Input: part model. Units: mm. Frame: model coordinates. A direction names the side the tool comes from. Round coordinates to 2 decimals unless told otherwise and drop trailing zeros. Order: outer loops, then holes, each group sorted by start corner. A loop starts at its lowest first (then second) coordinate and runs counter-clockwise, first axis right, second up.
Item 1: Cut plane A-A on z = 6.5. Output: boundary loops of the cut face in (x, y), then the cut area to 3 significant figures.
Item 2: First-contact query: pin 1 (1.2 mm diameter, centred on y = 3, z = 5, fed in from +X); pin 2 (5 mm diameter, centred on y = 2.25, z = 5, fed in from +X); pin 3 (2 mm diameter, centred on x = 12.5, y = 9, fed in from +Z). Flat tips, straight axial feed; report the tip coordinate or a pass-through.
Item 3: Cut plane B-B on x = 10.5. Output: boundary loops of the cut face in (y, z), then the cut area to 3 significant figures.
Item 4: Cut plane D-D on z = -5.75. Output: boundary loops of the cut face in (x, y).
Item 5: Mould query, pull axis Y, two halves, no side actions, for faces 1 (the flat face through (0, 12, 0)), 2 (the flat face through (9.25, 11.5, -6.8)), 3 (the cylindrical face through (12.7, 0.71, 6.64)). Classes: released by +Y, released by -Y, zero draft, split by the parting line, or undercut.
Item 6: Reachability of faces 4 (the cylindrical face through (12.7, 11.39, 6.54)), 5 (the flat face through (9.25, 0.5, 6.8)), 6 (the flat face through (9.25, 11, 0)), 7 (the flat face through (9.25, 6, -6)), 8 (the cylindrical face through (13.487, 5.324, 6.726)) from +Z, -Z, +X, -X, +Y, -Y: full face, straight path, thin tool, end or side. Return the list, or none.
Item 7: Cut plane C-C on y = 6. Output: boundary loops of the cut face in (x, z), then the cut area to 3 significant figures.
Item 8: Line query: L1, parallel to Y at x = 16, z = -6; L2, parallel to X at y = 5.5, z = 4.25; L3, parallel to X at y = 8, z = 4.5. Output: solid intervals per line, ascending.
```python
from build123d import *

# Parameters (mm, degrees)
SKETCH_1_W      = 18.5
SKETCH_1_H      = 14.5
EXTRUDE_1_DEPTH = 12
SKETCH_2_R      = 2.25
SKETCH_2_R_2    = 2
EXTRUDE_2_DEPTH = 7
SKETCH_4_R      = 1.5
EXTRUDE_3_DEPTH = 5.5
SKETCH_6_R      = 1
EXTRUDE_4_DEPTH = 3.5


with BuildPart() as part:
    # 스케치1 → 보스-돌출1 (new body)
    with BuildSketch(Plane(origin=(0, 0, 0), x_dir=(1, 0, 0), z_dir=(0, 1, 0))):
        Rectangle(SKETCH_1_W, SKETCH_1_H)
    extrude(amount=EXTRUDE_1_DEPTH)

    # 스케치2 → 보스-돌출2 (add)
    # profile 1 of 5: a face of its own
    with BuildSketch(Plane(origin=(9.25, 0, 0), x_dir=(0, 0, -1), z_dir=(1, 0, 0))):
        with Locations((-5, 9.75)):
            Circle(SKETCH_2_R)
        with Locations((-5, 9.75)):
            Circle(SKETCH_2_R_2, mode=Mode.SUBTRACT)
    # profile 2 of 5: a face of its own
    with BuildSketch(Plane(origin=(9.25, 0, 0), x_dir=(0, 0, -1), z_dir=(1, 0, 0))):
        with BuildLine():
            Line((2.75, 9.75), (-2.75, 9.75))
            ThreePointArc((-2.75, 9.75), (-3.409009742, 8.159009742), (-5, 7.5))
            Line((-5, 7.5), (-5, 4.5))
            ThreePointArc((-5, 4.5), (-3.409009742, 3.840990258), (-2.75, 2.25))
            Line((-2.75, 2.25), (2.75, 2.25))
            ThreePointArc((2.75, 2.25), (3.409009742, 3.840990258), (5, 4.5))
            Line((5, 4.5), (5, 7.5))
            ThreePointArc((5, 7.5), (3.409009742, 8.159009742), (2.75, 9.75))
        make_face()
    # profile 3 of 5: a face of its own
    with BuildSketch(Plane(origin=(9.25, 0, 0), x_dir=(0, 0, -1), z_dir=(1, 0, 0))):
        with Locations((5, 9.75)):
            Circle(SKETCH_2_R)
        with Locations((5, 9.75)):
            Circle(SKETCH_2_R_2, mode=Mode.SUBTRACT)
    # profile 4 of 5: a face of its own
    with BuildSketch(Plane(origin=(9.25, 0, 0), x_dir=(0, 0, -1), z_dir=(1, 0, 0))):
        with Locations((5, 2.25)):
            Circle(SKETCH_2_R)
        with Locations((5, 2.25)):
            Circle(SKETCH_2_R_2, mode=Mode.SUBTRACT)
    # profile 5 of 5: a face of its own
    with BuildSketch(Plane(origin=(9.25, 0, 0), x_dir=(0, 0, -1), z_dir=(1, 0, 0))):
        with Locations((-5, 2.25)):
            Circle(SKETCH_2_R)
        with Locations((-5, 2.25)):
            Circle(SKETCH_2_R_2, mode=Mode.SUBTRACT)
    extrude(amount=EXTRUDE_2_DEPTH)

    # 스케치4 → 보스-돌출3 (add)
    with BuildSketch(Plane(origin=(16.25, 0, 0), x_dir=(0, 0, -1), z_dir=(1, 0, 0))):
        with Locations((0, 6)):
            Circle(SKETCH_4_R)
    extrude(amount=EXTRUDE_3_DEPTH)

    # 스케치6 → 보스-돌출4 (add)
    with BuildSketch(Plane.XY.offset(5)):
        with Locations(Location((12.75, 6, 0), (0, 0, 180))):
            Circle(SKETCH_6_R)
    extrude(amount=EXTRUDE_4_DEPTH)


solid = part.part
```
From the geometry:
1. outline: (-9.25, 0) - (9.25, 0) - (9.25, 0.57) - (16.25, 0.57) - (16.25, 0.93) - (9.25, 0.93) - (9.25, 3.57) - (16.25, 3.57) - (16.25, 3.93) - (9.25, 3.93) - (9.25, 8.07) - (16.25, 8.07) - (16.25, 8.43) - (9.25, 8.43) - (9.25, 11.07) - (16.25, 11.07) - (16.25, 11.43) - (9.25, 11.43) - (9.25, 12) - (-9.25, 12) - close; circle Ø2 at (12.75, 6)
1. area: 235 mm2
2. pin 1: stops at x = 9.25
2. pin 2: stops at x = 16.25
2. pin 3: stops at z = 7.25
3. outline: (2.25, -2.75) arc R2.25 ccw (long way) to (4.5, -5) - (7.5, -5) arc R2.25 ccw (long way) to (9.75, -2.75) - (9.75, 2.75) arc R2.25 ccw (long way) to (7.5, 5) - (4.5, 5) arc R2.25 ccw (long way) to (2.25, 2.75) - close; hole circle Ø4 at (2.25, -5); hole circle Ø4 at (2.25, 5); hole circle Ø4 at (9.75, -5); hole circle Ø4 at (9.75, 5)
3. area: 72.4 mm2
4. outline: (-9.25, 0) - (9.25, 0) - (9.25, 0.13) - (16.25, 0.13) - (16.25, 0.4) - (9.25, 0.4) - (9.25, 4.1) - (16.25, 4.1) - (16.25, 4.37) - (9.25, 4.37) - (9.25, 7.63) - (16.25, 7.63) - (16.25, 7.9) - (9.25, 7.9) - (9.25, 11.6) - (16.25, 11.6) - (16.25, 11.87) - (9.25, 11.87) - (9.25, 12) - (-9.25, 12) - close
5. face 1: released by +Y
5. face 2: zero draft
5. face 3: undercut
6. face 4: +X
6. face 5: +Z, +X, -Y
6. face 6: +X, +Y
6. face 7: -Z, +X
6. face 8: +Z
7. outline: (-9.25, -7.25) - (9.25, -7.25) - (9.25, -5) - (16.25, -5) - (16.25, -1.5) - (21.75, -1.5) - (21.75, 1.5) - (16.25, 1.5) - (16.25, 5) - (13.75, 5) - (13.75, 8.5) - (11.75, 8.5) - (11.75, 5) - (9.25, 5) - (9.25, 7.25) - (-9.25, 7.25) - close
7. area: 362 mm2
8. L1: y = 0.23 to 0.52, 3.98 to 4.27, 7.73 to 8.02, 11.48 to 11.77
8. L2: x = -9.25 to 16.25
8. L3: x = -9.25 to 9.25
